Check sheet for the modelled part. Datum: model origin and axes. Units: mm. A direction names the side the tool comes from. Round coordinates to 2 decimals unless told otherwise and drop trailing zeros. Loops run counter-clockwise (first coordinate to the right, second up) from the corner with the lowest first, then second, coordinate; pieces in that order, holes last. Notation, with made-up numbers: M 88.5,-4 L 124.5,-4 A30 cw 124.5,26 Z; hole C 12,-40 d2. An arc over 180 degrees is marked long. Write item = value, one per line. Start each with the question number.
(1) Cross-section at C-C on x = 0. Record the boundary of the cut face in (y, z), plus the area to 3 significant figures.
(2) Set-up check for faces 1 (the face through (12.08, 1.48, 2.85)), 2 (the face through (-4.88, 4.97, -1.08)): record each of +Z, -Z, +X, -X, +Y, -Y from which the full face is reachable in a straight line by a thin tool's end or side.
(3) Cross-section at A-A on z = 0. Record the boundary of the cut face in (x, y).
(4) Mould release check, pull along Z, two halves, no side actions. Record for faces 3 (the face through (0.9, 5.03, 2.86)), 4 (the face through (0, 1.5, 18.5)), 5 (the face through (-4.164, 1.479, -6.086)): pulls with the +Z half, pulls with the -Z half, needs draft (parallel to the pull), parting line crosses it, or undercut.
(5) Go/stop test with flat-tipped pins: P1, Ø3.5, axis at x = 0, z = 0, coming from the +Y side; P2, Ø2, axis at x = -13.5, y = 2, coming from the -Z side; P3, Ø4, axis at x = -12, y = 4.5, coming from the -Z side. Record where each tip stops, or that it passes through.
(6) Cross-section at D-D on y = 6. Record the boundary of the cut face in (x, z).
(7) Scan lines: L1, parallel to X at y = 5.65, z = 0; L2, parallel to Y at x = 6.5, z = -3; L3, parallel to X at y = 1.25, z = -13. Record each from-to range of solid material in increasing order. Write a range as from..to.
(8) Cross-section at B-B on y = 1.5. Record the boundary of the cut face in (x, z), plus the area to 3 significant figures.
from build123d import *

# Parameters (mm, degrees)
BOSS_EXTRUDE1_DEPTH = 3
SKETCH2_R           = 5
BOSS_EXTRUDE2_DEPTH = 4
SKETCH3_R           = 3
CUT_EXTRUDE1_DEPTH  = 4
FILLET1_R           = 5


with BuildPart() as part:
    # Sketch1 → Boss-Extrude1 (new body)
    with BuildSketch(Plane(origin=(0, 0, 0), x_dir=(1, 0, 0), z_dir=(0, 1, 0))):
        with BuildLine():
            Line((-1.966664332, 16.863636364), (-4.025937287, 5.726415018))
            ThreePointArc((-4.025937287, 5.726415018), (-4.949747468, 4.949747468), (-5.726415018, 4.025937287))
            Line((-5.726415018, 4.025937287), (-16.863636364, 1.966664332))
            ThreePointArc((-16.863636364, 1.966664332), (-18.5, 0), (-16.863636364, -1.966664332))
            Line((-16.863636364, -1.966664332), (-5.726415018, -4.025937287))
            ThreePointArc((-5.726415018, -4.025937287), (-4.949747468, -4.949747468), (-4.025937287, -5.726415018))
            Line((-4.025937287, -5.726415018), (-1.966664332, -16.863636364))
            ThreePointArc((-1.966664332, -16.863636364), (0, -18.5), (1.966664332, -16.863636364))
            Line((1.966664332, -16.863636364), (4.025937287, -5.726415018))
            ThreePointArc((4.025937287, -5.726415018), (4.949747468, -4.949747468), (5.726415018, -4.025937287))
            Line((5.726415018, -4.025937287), (16.863636364, -1.966664332))
            ThreePointArc((16.863636364, -1.966664332), (18.5, 0), (16.863636364, 1.966664332))
            Line((16.863636364, 1.966664332), (5.726415018, 4.025937287))
            ThreePointArc((5.726415018, 4.025937287), (4.949747468, 4.949747468), (4.025937287, 5.726415018))
            Line((4.025937287, 5.726415018), (1.966664332, 16.863636364))
            ThreePointArc((1.966664332, 16.863636364), (0, 18.5), (-1.966664332, 16.863636364))
        make_face()
    extrude(amount=BOSS_EXTRUDE1_DEPTH)

    # Sketch2 → Boss-Extrude2 (add)
    with BuildSketch(Plane(origin=(0, 3, 0), x_dir=(1, 0, 0), z_dir=(0, 1, 0))):
        with Locations(Location((0, 0, 0), (0, 0, 270))):
            Circle(SKETCH2_R)
    extrude(amount=BOSS_EXTRUDE2_DEPTH)

    # Sketch3 → Cut-Extrude1 (cut)
    with BuildSketch(Plane(origin=(0, 7, 0), x_dir=(1, 0, 0), z_dir=(0, 1, 0))):
        with Locations(Location((0, 0, 0), (0, 0, 270))):
            Circle(SKETCH3_R)
    extrude(amount=-CUT_EXTRUDE1_DEPTH, mode=Mode.SUBTRACT)

    # Fillet1
    # the kernel refuses this fillet: 5 mm, written as the material it adds along each edge
    with BuildSketch(Plane(origin=(5.726415018, 0, 4.025937287), x_dir=(0.983332166035634, 0, -0.18181818181817894), z_dir=(0, 1, 0))) as fillet1_piece_1:
        with BuildLine():
            CenterArc((1.734270095, -5), FILLET1_R, 90, 33.557309762)
            ThreePointArc((-1.029583897, -0.833333333), (-0.495036767, -0.441074207), (0, 0))
            Line((0, 0), (1.734270095, 0))
        make_face()
    extrude(amount=3)
    with BuildSketch(Plane(origin=(4.025937287, 0, 5.726415018), x_dir=(0.7599749646341246, 0, -0.6499523468142576), z_dir=(0, 1, 0))) as fillet1_piece_2:
        with BuildLine():
            CenterArc((1.797631616, -4.977571028), FILLET1_R, 95.428999418, 33.557309762)
            Line((-1.348041755, -1.091089451), (0, 0))
            ThreePointArc((0, 0), (0.662285332, -0.031400561), (1.324570664, 0))
        make_face()
    extrude(amount=3)
    with BuildSketch(Plane(origin=(-4.025937287, 0, 5.726415018), x_dir=(-0.7599749646342022, 0, -0.6499523468141668), z_dir=(0, 1, 0)), Plane(origin=(-5.726415018, 0, -4.025937287), x_dir=(0.6499523468141845, 0, -0.7599749646341871), z_dir=(0, 1, 0)), Plane(origin=(4.025937287, 0, -5.726415018), x_dir=(0.7599749646341224, 0, 0.6499523468142602), z_dir=(0, 1, 0))) as fillet1_piece_3:
        with BuildLine():
            CenterArc((1.797631616, 4.977571028), FILLET1_R, 231.01369082, 33.557309762)
            Line((-1.348041755, 1.091089451), (0, 0))
            ThreePointArc((0, 0), (0.662285332, 0.031400561), (1.324570664, 0))
        make_face()
    extrude(amount=3)
    with BuildSketch(Plane(origin=(-5.726415018, 0, 4.025937287), x_dir=(-0.9833321660356334, 0, -0.18181818181818182), z_dir=(0, 1, 0)), Plane(origin=(-4.025937287, 0, -5.726415018), x_dir=(0.1818181818181817, 0, -0.9833321660356334), z_dir=(0, 1, 0)), Plane(origin=(5.726415018, 0, -4.025937287), x_dir=(0.9833321660356329, 0, 0.1818181818181846), z_dir=(0, 1, 0))) as fillet1_piece_4:
        with BuildLine():
            CenterArc((1.734270095, 5), FILLET1_R, 236.442690238, 33.557309762)
            ThreePointArc((-1.029583897, 0.833333333), (-0.495036767, 0.441074207), (0, 0))
            Line((0, 0), (1.734270095, 0))
        make_face()
    extrude(amount=3)


solid = part.part
Result:
q1.outline = M 0,-18.5 L 3,-18.5 L 3,-5 L 7,-5 L 7,-3 L 3,-3 L 3,3 L 7,3 L 7,5 L 3,5 L 3,18.5 L 0,18.5 Z
q1.area = 127 mm^2
q2.face_1 = +Z, +X, +Y, -Y
q2.face_2 = +Y
q3.outline = M -18.5,0 L 18.5,0 L 18.5,3 L 5,3 L 5,7 L 3,7 L 3,3 L -3,3 L -3,7 L -5,7 L -5,3 L -18.5,3 Z
q4.face_3 = undercut
q4.face_4 = pulls with the +Z half
q4.face_5 = pulls with the -Z half
q5.P1 = 3
q5.P2 = -2.77
q5.P3 = -3.11
q6.outline = C 0,0 d10; hole C 0,0 d6
q7.L1 = -5..-3, 3..5
q7.L2 = 0..3
q7.L3 = -2.68..2.68
q8.outline = M -16.86,-1.97 L -7.43,-3.71 A5 cw -4.95,-4.95 A5 cw -3.71,-7.43 L -1.97,-16.86 A2 ccw 1.97,-16.86 L 3.71,-7.43 A5 cw 4.95,-4.95 A5 cw 7.43,-3.71 L 16.86,-1.97 A2 ccw 16.86,1.97 L 7.43,3.71 A5 cw 4.95,4.95 A5 cw 3.71,7.43 L 1.97,16.86 A2 ccw -1.97,16.86 L -3.71,7.43 A5 cw -4.95,4.95 A5 cw -7.43,3.71 L -16.86,1.97 A2 ccw Z
q8.area = 415 mm^2
